Source: CAD feature listing. Evaluate the final solid. Frame: model axes, mm. Round coordinates to 2 decimals unless told otherwise and drop trailing zeros. Order: outer loops, then holes, each group sorted by start corner. A loop starts at its lowest first (then second) coordinate and runs counter-clockwise, first axis right, second up. Notation, with made-up numbers: M 5.5,63.5 L 46.5,63.5 A9 cw 46.5,68.5 Z; hole C -40,37 d7. An arc over 180 degrees is marked long. Answer as CSV lines item,"result". Start each with the question number.
Item 1: Section query B-B on x = -804.5. Return the cut outline in (y, z).
Item 2: Line query: line 1 (Y direction, x = -950, z = 12.25); line 2 (X direction, y = 26.5, z = 5); line 3 (X direction, y = 19, z = 2.25). Output: solid intervals per line, ascending. Write a range as [from, to].
Item 3: Section query A-A on z = 7.75. Return the cut outline in (x, y), plus the area to 3 significant figures.
Item 4: First-contact query: P1, Ø5, axis at x = -259, z = 10, coming from the +Y side; P2, Ø10, axis at x = -991, z = 7.5, coming from the +Y side; P3, Ø6, axis at x = -1454.5, z = 2, coming from the +Y side. Flat tips, straight axial feed; report the tip coordinate or a pass-through.
Item 5: Pull-direction query (Y, two-part tool) for faces 1 (the face through (-1418.35, -50.28, 9.86)), 2 (the face through (-974, -18, 10)), 3 (the face through (-361.237, 47.745, 9.86)), 4 (the face through (-936, -30, 20)); classes: +Y half, -Y half, draft (parallel to the pull), parting line (faces both ways), or undercut.
Item 6: Section query C-C on x = -1762. Return the cut outline in (y, z), plus the area to 3 significant figures.
from build123d import *

# Parameters (mm, degrees)
SKIZZE1_R                       = 30
SKIZZE1_R_2                     = 6
AUFSATZ_LINEAR_AUSTRAGEN1_DEPTH = 20


with BuildPart() as part:
    # Skizze1 → Aufsatz-Linear austragen1 (new body)
    with BuildSketch(Plane.XY):
        with BuildLine():
            Line((-950, 70), (-712.5, 65))
            Line((-712.5, 65), (0, 30))
            ThreePointArc((0, 30), (30, 0), (0, -30))
            Line((0, -30), (-712.5, -65))
            Line((-712.5, -65), (-950, -70))
            Line((-950, -70), (-1900, -30))
            ThreePointArc((-1900, -30), (-1930, 0), (-1900, 30))
            Line((-1900, 30), (-950, 70))
        make_face()
        with Locations((-950, 0)):
            Circle(SKIZZE1_R, mode=Mode.SUBTRACT)
        with Locations((-712.5, 0)):
            Circle(SKIZZE1_R, mode=Mode.SUBTRACT)
        with Locations((-1900, 0)):
            Circle(SKIZZE1_R_2, mode=Mode.SUBTRACT)
        Circle(SKIZZE1_R_2, mode=Mode.SUBTRACT)
    extrude(amount=AUFSATZ_LINEAR_AUSTRAGEN1_DEPTH)


solid = part.part
Results:
1,outline,"M -66.94,0 L 66.94,0 L 66.94,20 L -66.94,20 Z"
2,line 1,"[-70, -30], [30, 70]"
2,line 2,"[-1914.06, -964.06], [-935.94, -726.56], [-698.44, 14.06]"
2,line 3,"[-1923.22, -973.22], [-926.78, -735.72], [-689.28, 23.22]"
3,outline,"M -1900,-30 L -950,-70 L -712.5,-65 L 0,-30 A30 ccw 0,30 L -712.5,65 L -950,70 L -1900,30 A30 ccw Z; hole C -1900,0 d12; hole C -950,0 d60; hole C -712.5,0 d60; hole C 0,0 d12"
3,area,"192,000 mm^2"
4,P1,"y = 42.85"
4,P2,"y = 68.48"
4,P3,"y = 48.88"
5,face 1,"-Y half"
5,face 2,"undercut"
5,face 3,"+Y half"
5,face 4,"draft"
6,outline,"M -35.81,0 L 35.81,0 L 35.81,20 L -35.81,20 Z"
6,area,"1,430 mm^2"
